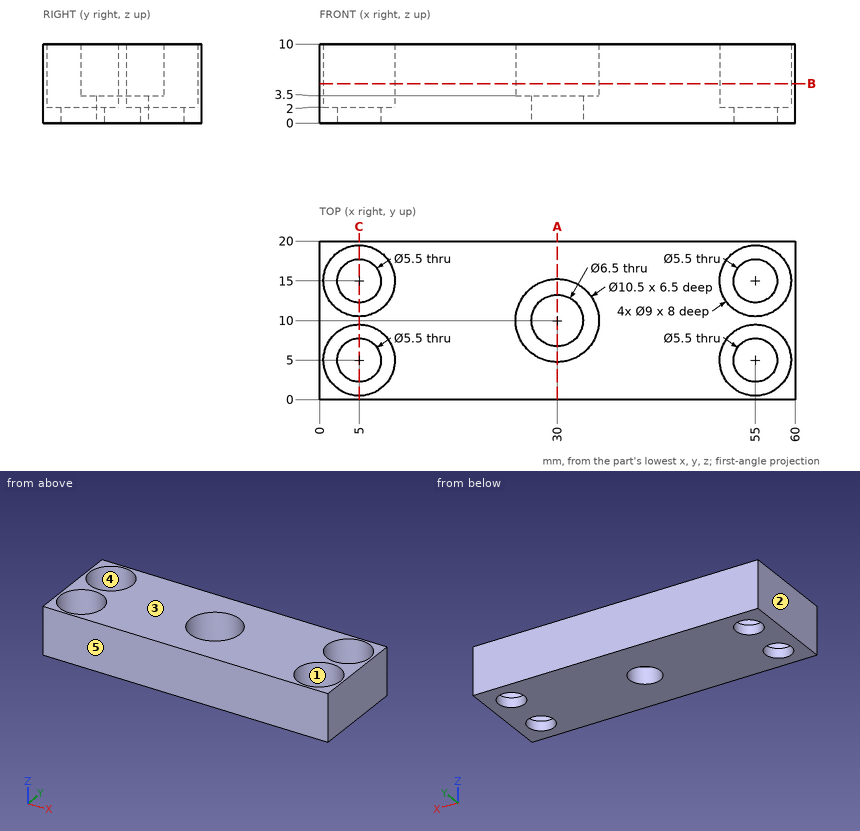
Study the drawing (mm; zero at the part's minimum x, y, z) and answer. A direction names the side the tool comes from. Coordinates: 2 decimals unless noted, no trailing zeros. Write each loop counter-clockwise with the first axis right and the second up, starting at its lowest first coordinate (ties: lowest second). Pieces come first, ordered by that corner, then holes.
Q1. Section B-B, the plane z = 5 is taken. Write down the section's boundary in (x, y), then the cut area to 3 significant figures.
Returned:
outline: (0, 0) - (60, 0) - (60, 20) - (0, 20) - close; hole circle Ø9 at (5, 5); hole circle Ø9 at (5, 15); hole circle Ø10.5 at (30, 10); hole circle Ø9 at (55, 5); hole circle Ø9 at (55, 15)
area: 859 mm2
Q2. Given P1, Ø8, axis at x = 41.5, y = 2, coming from the -Z side; P2, Ø2.5, axis at x = 56.5, y = 15.5, coming from the +Z side; P3, Ø3, axis at x = 28.5, y = 11, coming from the +Z side, each flat-ended and moving along its own axis, determine where each tip first touches the part or whether it passes through.
Returned:
P1: stops at z = 0
P2: stops at z = 2
P3: stops at z = 3.5
Q3. The mould has two halves that part along X. Classify the marked faces 1, 2 and 3: released by +X, released by -X, zero draft, split by the parting line, or undercut.
Returned:
face 1: undercut
face 2: released by -X
face 3: zero draft
Q4. Section C-C, the plane x = 5 is taken. Write down the section's boundary in (y, z), then the cut area to 3 significant figures.
Returned:
outline: (0, 0) - (2.25, 0) - (2.25, 2) - (0.5, 2) - (0.5, 10) - (0, 10) - close; (7.75, 0) - (12.25, 0) - (12.25, 2) - (10.5, 2) - (10.5, 10) - (9.5, 10) - (9.5, 2) - (7.75, 2) - close; (17.75, 0) - (20, 0) - (20, 10) - (19.5, 10) - (19.5, 2) - (17.75, 2) - close
area: 34.0 mm2
Q5. Section A-A, the plane x = 30 is taken. Write down the section's boundary in (y, z).
Returned:
outline: (0, 0) - (6.75, 0) - (6.75, 3.5) - (4.75, 3.5) - (4.75, 10) - (0, 10) - close; (13.25, 0) - (20, 0) - (20, 10) - (15.25, 10) - (15.25, 3.5) - (13.25, 3.5) - close
Q6. Which of the six approach directions +Z, -Z, +X, -X, +Y, -Y give full straight-line access (tool end or side, diameter ignored) to the marked faces 4 and 5?
Returned:
face 4: +Z
face 5: +Z, -Z, +X, -X, -Y
Q7. Find the intervals of material crossed by line 1 along X through (y, z) = (5, 0.7); line 2 along Y through (x, z) = (5, 0.85); line 3 along X through (y, z) = (15, 3), in increasing order.
Returned:
line 1: x = 0 to 2.25, 7.75 to 52.25, 57.75 to 60
line 2: y = 0 to 2.25, 7.75 to 12.25, 17.75 to 20
line 3: x = 0 to 0.5, 9.5 to 50.5, 59.5 to 60
